Design review of the part built by this model. Coordinates are the model's own, in mm. A direction names the side the tool comes from. Coordinates: 2 decimals unless noted, no trailing zeros. Loops run counter-clockwise (first coordinate to the right, second up) from the corner with the lowest first, then second, coordinate; pieces in that order, holes last. Notation, with made-up numbers: (-18.75, -20) -> (-6.75, -20) arc R21 cw to (-6.75, 19) -> close; hole circle Ø1 at (-12, 61.5). An arc over 180 degrees is marked (long way). Answer in a Markdown table with one row per item.
Solid Edge part; units mm, degrees
sketch "Sketch1" plane through (0, 0, 0) normal (0, 0, 1) x (1, 0, 0)
  line L0 (3, 0) -> (3, 12)
  line L1 (0, 12) -> (3, 12)
  line L2 (0, 0) -> (0, 12)
  line L3 (0, 0) -> (0, -6)
  line L4 (0, -6) -> (5, -6)
  line L5 (5, -6) -> (5, 0)
  line L6 (5, 0) -> (3, 0)
revolve "RevolvedProtrusion1" add sketch "Sketch1" angle 360 about axis through (0, 0, 0) along (0, 1, 0)
sketch "Sketch2" plane through (0, 0, 0) normal (1, 0, 0) x (0, 1, 0)
  line L0 (-6, 3.3615) -> (-3, 3.3615)
  line L1 (-1.0592, 0) -> (-3, 3.3615)
  line L2 (-6, 0) -> (-1.0592, 0)
  line L3 (-6, 0) -> (-6, 3.3615)
revolve "RevolvedCutout1" cut sketch "Sketch2" angle 360 about axis through (0, -4.5, 0) along (0, 1, 0)
sketch "Sketch3" plane through (0, -6, 0) normal (0, -1, 0) x (0, 0, 1)
  circle A0 centre (0, 0) radius 3.3615
  line L0 (-2.5, -1.4434) -> (0, -2.8868)
  line L1 (0, -2.8868) -> (2.5, -1.4434)
  line L2 (2.5, -1.4434) -> (2.5, 1.4434)
  line L3 (2.5, 1.4434) -> (0, 2.8868)
  line L4 (0, 2.8868) -> (-2.5, 1.4434)
  line L5 (-2.5, 1.4434) -> (-2.5, -1.4434)
extrude "Protrusion1" add sketch "Sketch3" against normal up to next
sketch "Sketch4" plane through (0, 0, 0) normal (0, 0, 1) x (1, 0, 0)
  line L0 (-2.8868, -6) -> (0, -6)
  line L1 (0, -6) -> (0, -5.2265)
  line L2 (0, -5.2265) -> (-2.8868, -6)
revolve "RevolvedCutout2" cut sketch "Sketch4" angle 360 about axis through (0, -4.5, 0) along (0, 1, 0)
fillet "Round1" radius 0.25 1 edges at (0, 0, -3)
fillet "Round2" radius 0.5 1 edges at (0, -6, -5)
chamfer "倒斜角_2" distance 0.4 angle 45 1 edges at (0, 12, -3)
cosmetic_thread "螺纹_3" thread depth 9.6
(1) Take a section at A-A on y = 8. Give the boundary of the cut face in (x, z).
Evaluation:
| item | result |
|---|---|
| outline | circle Ø6 at (0, 0) |
(2) To check wall thickness, follow probe 1 along Y at (x, z) = (3.75, -1.25); probe 2 along X at (y, z) = (-3.5, -2.25); probe 3 along X at (y, z) = (-4.5, 0.5). State the ranges of each line that lie inside material, in increasing order.
Evaluation:
| item | result |
|---|---|
| probe 1 | y = -6 to 0 |
| probe 2 | x = -4.47 to -1.59, 1.59 to 4.47 |
| probe 3 | x = -4.97 to -2.6, 2.6 to 4.97 |
(3) Draft analysis for pull direction X (two halves, no side actions). For faces 1 (the conical face through (0.16, -1.163, 0.083)), 2 (the cylindrical face through (-3, 6, 0)), 3 (the flat face through (3.3, 0, 1)), state which applies: pulls with the +X half, pulls with the -X half, needs draft (parallel to the pull), parting line crosses it, or undercut.
Evaluation:
| item | result |
|---|---|
| face 1 | undercut |
| face 2 | parting line crosses it |
| face 3 | needs draft |
(4) Tool access review of faces 4 (the cylindrical face through (-1.08, -2.71, 4.88)), 5 (the flat face through (-2.175, -4.276, -1.233)): name each direction out of +Z, -Z, +X, -X, +Y, -Y from which nothing blocks a thin tool from reaching the whole face with its end or side.
Evaluation:
| item | result |
|---|---|
| face 4 | +Y, -Y |
| face 5 | -Y |
(5) For pin 1 (1 mm diameter, centred on x = 2, y = 7, fed in from -Z); pin 2 (3 mm diameter, centred on x = 2, y = 5.5, fed in from -Z); pin 3 (2 mm diameter, centred on y = 10, z = -2.5, fed in from -X), all flat-tipped, find the tip position at first contact; note any pin that passes through.
Evaluation:
| item | result |
|---|---|
| pin 1 | stops at z = -2.6 |
| pin 2 | stops at z = -2.96 |
| pin 3 | stops at x = -2.6 |
